Model file for the job. Use its own axes, mm. A direction names the side the tool comes from. Give positions to 0.01 mm unless a question says otherwise; leave off trailing zeros. Loops run counter-clockwise (first coordinate to the right, second up) from the corner with the lowest first, then second, coordinate; pieces in that order, holes last. Notation, with made-up numbers: (-20.75, -33.75) - (24.25, -33.75) arc R22 cw to (24.25, -13.75) - close; hole circle Ø7 at (42, -19.75). An arc over 180 degrees is marked (long way). Use a Markdown table: item, result.
Autodesk Inventor part; units mm, degrees
ref_plane "YZ Plane" through (0, 0, 0) normal (1, 0, 0) x (0, 1, 0)
ref_plane "XZ Plane" through (0, 0, 0) normal (0, 1, 0) x (-1, 0, 0)
ref_plane "XY Plane" through (0, 0, 0) normal (0, 0, 1) x (1, 0, 0)
sketch "Sketch1" plane through (0, 0, 0) normal (0, 0, 1) x (1, 0, 0)
  line L0 (1.5875, 3.175) -> (7.9375, 3.175)
  line L1 (7.9375, 3.175) -> (7.9375, 0)
  line L2 (7.9375, 0) -> (1.5875, 0)
  line L3 (1.5875, 0) -> (1.5875, 3.175)
  line L4 (-7.9375, 3.175) -> (-1.5875, 3.175)
  line L5 (-1.5875, 3.175) -> (-1.5875, 0)
  line L6 (-1.5875, 0) -> (-7.9375, 0)
  line L7 (-7.9375, 0) -> (-7.9375, 3.175)
  line L8 (7.9375, 0) -> (4.7625, 0)
  line L9 (4.7625, 0) -> (4.7625, -3.175)
  line L10 (4.7625, -3.175) -> (7.9375, -3.175)
  line L11 (7.9375, -3.175) -> (7.9375, 0)
  line L12 (-7.9375, 0) -> (-4.7625, 0)
  line L13 (-4.7625, 0) -> (-4.7625, -3.175)
  line L14 (-4.7625, -3.175) -> (-7.9375, -3.175)
  line L15 (-7.9375, -3.175) -> (-7.9375, 0)
  line L16 (-4.7625, -3.175) -> (-1.5875, -6.35)
  line L17 (-1.5875, -6.35) -> (1.5875, -6.35)
  line L18 (1.5875, -6.35) -> (4.7625, -3.175)
  line L19 (7.9375, -3.175) -> (1.5875, -9.525)
  line L20 (1.5875, -9.525) -> (-1.5875, -9.525)
  line L21 (-1.5875, -9.525) -> (-7.9375, -3.175)
  line L22 (-7.9375, -3.175) -> (-4.7625, -3.175)
  point P0 (0, 0)
  dimension "d0" = 6.35
  dimension "d1" = 3.175
  dimension "d2" = 1.5875
  dimension "d3" = 3.175
  dimension "d4" = 6.35
  dimension "d5" = 3.175
  dimension "d6" = 3.175
  dimension "d7" = 4.7625
  dimension "d8" = 4.7625
  dimension "d9" = 3.175
  dimension "d10" = 3.175
  dimension "d11" = 135
  dimension "d12" = 3.175
extrude "Extrusion1" add sketch "Sketch1" against normal blind 50.8
sketch "Sketch2" plane through (7.9375, -3.175, 0) normal (1, 0, 0) x (0, 0, -1)
  line L0 (0, 3.175) -> (50.8, 3.175)
  line L1 (3.175, 3.175) -> (6.35, 3.175)
  line L2 (6.35, 3.175) -> (6.35, -6.35)
  line L3 (6.35, -6.35) -> (3.175, -6.35)
  line L4 (3.175, -6.35) -> (3.175, 3.175)
  line L5 (0, 0) -> (0, 6.35)
  line L6 (9.525, 3.175) -> (12.7, 3.175)
  line L7 (12.7, 3.175) -> (12.7, -6.35)
  line L8 (12.7, -6.35) -> (9.525, -6.35)
  line L9 (9.525, -6.35) -> (9.525, 3.175)
  line L10 (15.875, 3.175) -> (19.05, 3.175)
  line L11 (19.05, 3.175) -> (19.05, -6.35)
  line L12 (19.05, -6.35) -> (15.875, -6.35)
  line L13 (15.875, -6.35) -> (15.875, 3.175)
  line L14 (22.225, 3.175) -> (25.4, 3.175)
  line L15 (25.4, 3.175) -> (25.4, -6.35)
  line L16 (25.4, -6.35) -> (22.225, -6.35)
  line L17 (22.225, -6.35) -> (22.225, 3.175)
  line L18 (28.575, 3.175) -> (31.75, 3.175)
  line L19 (31.75, 3.175) -> (31.75, -6.35)
  line L20 (31.75, -6.35) -> (28.575, -6.35)
  line L21 (28.575, -6.35) -> (28.575, 3.175)
  line L22 (34.925, 3.175) -> (38.1, 3.175)
  line L23 (38.1, 3.175) -> (38.1, -6.35)
  line L24 (38.1, -6.35) -> (34.925, -6.35)
  line L25 (34.925, -6.35) -> (34.925, 3.175)
  line L26 (41.275, 3.175) -> (44.45, 3.175)
  line L27 (44.45, 3.175) -> (44.45, -6.35)
  line L28 (44.45, -6.35) -> (41.275, -6.35)
  line L29 (41.275, -6.35) -> (41.275, 3.175)
  line L30 (47.625, 3.175) -> (50.8, 3.175)
  line L31 (50.8, 3.175) -> (50.8, -6.35)
  line L32 (50.8, -6.35) -> (47.625, -6.35)
  line L33 (47.625, -6.35) -> (47.625, 3.175)
  dimension "d15" = 3.175
  dimension "d16" = 3.175
  dimension "d17" = 9.525
  dimension "d18" = 3.175
  dimension "d19" = 3.175
  dimension "d20" = 3.175
  dimension "d21" = 3.175
  dimension "d22" = 3.175
  dimension "d23" = 3.175
  dimension "d24" = 3.175
  dimension "d25" = 3.175
  dimension "d26" = 3.175
  dimension "d27" = 3.175
  dimension "d28" = 3.175
  dimension "d29" = 3.175
  dimension "d30" = 3.175
  dimension "d31" = 3.175
extrude "Extrusion2" cut sketch "Sketch2" against normal blind 6.35
sketch "Sketch3" plane through (-7.9375, -3.175, 0) normal (-1, 0, 0) x (0, 0, 1)
  line L0 (-3.175, 3.175) -> (-3.175, 3.175)
  line L1 (-50.8, 3.175) -> (-47.625, 3.175)
  line L2 (-47.625, 3.175) -> (-47.625, -6.35)
  line L3 (-47.625, -6.35) -> (-50.8, -6.35)
  line L4 (-50.8, -6.35) -> (-50.8, 3.175)
  line L5 (-44.45, 3.175) -> (-41.275, 3.175)
  line L6 (-41.275, 3.175) -> (-41.275, -6.35)
  line L7 (-41.275, -6.35) -> (-44.45, -6.35)
  line L8 (-44.45, -6.35) -> (-44.45, 3.175)
  line L9 (-38.1, 3.175) -> (-34.925, 3.175)
  line L10 (-34.925, 3.175) -> (-34.925, -6.35)
  line L11 (-34.925, -6.35) -> (-38.1, -6.35)
  line L12 (-38.1, -6.35) -> (-38.1, 3.175)
  line L13 (-31.75, 3.175) -> (-28.575, 3.175)
  line L14 (-28.575, 3.175) -> (-28.575, -6.35)
  line L15 (-28.575, -6.35) -> (-31.75, -6.35)
  line L16 (-31.75, -6.35) -> (-31.75, 3.175)
  line L17 (-25.4, 3.175) -> (-22.225, 3.175)
  line L18 (-22.225, 3.175) -> (-22.225, -6.35)
  line L19 (-22.225, -6.35) -> (-25.4, -6.35)
  line L20 (-25.4, -6.35) -> (-25.4, 3.175)
  line L21 (-19.05, 3.175) -> (-15.875, 3.175)
  line L22 (-15.875, 3.175) -> (-15.875, -6.35)
  line L23 (-15.875, -6.35) -> (-19.05, -6.35)
  line L24 (-19.05, -6.35) -> (-19.05, 3.175)
  line L25 (-12.7, 3.175) -> (-9.525, 3.175)
  line L26 (-9.525, 3.175) -> (-9.525, -6.35)
  line L27 (-9.525, -6.35) -> (-12.7, -6.35)
  line L28 (-12.7, -6.35) -> (-12.7, 3.175)
  line L29 (-6.35, -6.35) -> (-6.35, 3.175)
  line L30 (-6.35, 3.175) -> (-3.175, 3.175)
  line L31 (-3.175, 3.175) -> (-3.175, -6.35)
  line L32 (-3.175, -6.35) -> (-6.35, -6.35)
  point P0 (0, 3.175)
  point P1 (-3.175, 0)
  dimension "d34" = 3.175
  dimension "d35" = 9.525
  dimension "d36" = 3.175
  dimension "d37" = 3.175
  dimension "d38" = 3.175
  dimension "d39" = 3.175
  dimension "d40" = 3.175
  dimension "d41" = 3.175
  dimension "d42" = 3.175
  dimension "d43" = 3.175
  dimension "d44" = 3.175
  dimension "d45" = 3.175
  dimension "d46" = 3.175
  dimension "d47" = 3.175
  dimension "d48" = 3.175
  dimension "d49" = 3.175
extrude "Extrusion3" cut sketch "Sketch3" against normal blind 6.35
sketch "Sketch4" plane through (-7.9375, 3.175, 0) normal (0, 1, 0) x (1, 0, 0)
  circle A0 centre (7.9375, 25.4) radius 9.525
  point P0 (7.9375, 0)
  dimension "d52" = 19.05
extrude "Extrusion4" add sketch "Sketch4" against normal blind 12.7
sketch "Sketch5" plane through (-7.9375, 3.175, 0) normal (0, 1, 0) x (1, 0, 0)
  arc A0 (6.35, 34.7918) -> (6.35, 16.0082) centre (7.9375, 25.4) ccw
  circle A1 centre (7.9375, 25.4) radius 3.4036
  point P0 (7.9375, 0)
  dimension "d55" = 6.8072
extrude "Extrusion5" cut sketch "Sketch5" against normal blind 12.7
sketch "Sketch6" plane through (0, 0, 0) normal (0, 0, 1) x (1, 0, 0)
  line L0 (-1.5875, 3.175) -> (-1.5875, 0)
  line L1 (-1.5875, 3.175) -> (1.5875, 3.175)
  line L2 (1.5875, 3.175) -> (1.5875, -3.175)
  line L3 (1.5875, -3.175) -> (-1.5875, -3.175)
  line L4 (-1.5875, -3.175) -> (-1.5875, 3.175)
  line L5 (-4.7625, -3.175) -> (-4.7625, 0)
  line L6 (-4.7625, 0) -> (4.7625, 0)
  line L7 (4.7625, 0) -> (4.7625, -3.175)
  line L8 (4.7625, -3.175) -> (-4.7625, -3.175)
  line L9 (-4.7625, -3.175) -> (-4.7625, 0)
  point P0 (0, 0)
extrude "Extrusion6" cut sketch "Sketch6" against normal blind 19.05
sketch "Sketch7" plane through (0, 0, -50.8) normal (0, 0, -1) x (-1, 0, 0)
  line L0 (-1.5875, 3.175) -> (-1.5875, 0)
  line L1 (-1.5875, 3.175) -> (1.5875, 3.175)
  line L2 (1.5875, 3.175) -> (1.5875, -3.175)
  line L3 (1.5875, -3.175) -> (-1.5875, -3.175)
  line L4 (-1.5875, -3.175) -> (-1.5875, 3.175)
  line L5 (-4.7625, -3.175) -> (-4.7625, 0)
  line L6 (-4.7625, 0) -> (4.7625, 0)
  line L7 (4.7625, 0) -> (4.7625, -3.175)
  line L8 (4.7625, -3.175) -> (-4.7625, -3.175)
  line L9 (-4.7625, -3.175) -> (-4.7625, 0)
  point P0 (0, 0)
  point P1 (0, 0)
extrude "Extrusion7" cut sketch "Sketch7" against normal blind 19.05
sketch "Sketch9" plane through (0, 0, 0) normal (0, 0, 1) x (1, 0, 0)
  line L0 (4.7625, 0) -> (1.5875, 0)
  line L1 (4.7625, -3.175) -> (4.7625, 0)
  line L2 (4.7625, 0) -> (4.7625, -3.175)
  line L3 (1.5875, -6.35) -> (4.7625, -3.175)
  line L4 (4.7625, -3.175) -> (1.5875, -6.35)
  line L5 (-1.5875, -6.35) -> (1.5875, -6.35)
  line L6 (1.5875, -6.35) -> (-1.5875, -6.35)
  line L7 (-1.5875, -6.35) -> (-4.7625, -3.175)
  line L8 (-1.5875, -6.35) -> (-4.7625, -3.175)
  line L9 (-4.7625, -3.175) -> (-4.7625, 0)
  line L10 (-7.9375, 0) -> (-4.7625, 0)
  line L11 (-4.7625, 0) -> (-7.9375, 0)
  line L12 (-7.9375, 0) -> (-7.9375, -3.175)
  line L13 (-7.9375, -3.175) -> (-1.5875, -9.525)
  line L14 (-7.0995, -4.013) -> (-7.9375, -3.175)
  line L15 (-1.5875, -9.525) -> (1.5875, -9.525)
  line L16 (-1.5875, -9.525) -> (1.5875, -9.525)
  line L17 (7.9375, -3.175) -> (1.5875, -9.525)
  line L18 (1.5875, -9.525) -> (7.9375, -3.175)
  line L19 (7.9375, 0) -> (7.9375, -3.175)
  line L20 (7.9375, -3.175) -> (7.9375, 0)
  line L21 (7.9375, 0) -> (4.7625, 0)
  point P0 (0, 0)
extrude "Extrusion8" add sketch "Sketch9" against normal blind 50.8
sketch "Sketch12" plane through (7.9375, -3.175, 0) normal (1, 0, 0) x (0, 0, -1)
  line L0 (3.175, 3.175) -> (6.35, 3.175)
  line L1 (0, 3.175) -> (19.05, 3.175)
  line L2 (0, 0) -> (17.1511, 0)
  line L3 (6.35, 3.175) -> (3.175, 0)
  line L4 (3.175, 0) -> (3.175, 3.175)
  line L5 (0, 0) -> (0, 6.35)
  line L6 (9.525, 3.175) -> (3.175, -3.175)
  line L7 (3.175, -3.175) -> (6.35, -3.175)
  line L8 (6.35, -3.175) -> (12.7, 3.175)
  line L9 (0, 3.175) -> (19.05, 3.175)
  dimension "d67" = 3.175
properties part number "Basic_rail2"
(1) Slice it at A-A, the plane x = 0. Write the cut outline in (y, z) (3 decimals).
Computed:
| item | result |
|---|---|
| outline | (-9.525, -50.8) - (-6.35, -50.8) - (-6.35, -34.925) - (-3.175, -34.925) - (-3.175, -31.75) - (3.175, -31.75) - (3.175, -28.804) - (-6.35, -28.804) - (-6.35, -21.996) - (3.175, -21.996) - (3.175, -19.05) - (-3.175, -19.05) - (-3.175, -15.875) - (-6.35, -15.875) - (-6.35, 0) - (-9.525, 0) - close |
(2) Mould opens along Z. For faces 1 (the flat face through (-4.762, -2, -9)), 2 (the cylindrical face through (-3.403, -8.804, -25.452)), 3 (the cylindrical face through (-9.523, -4.497, -25.587)) say: pulls with the +Z half, pulls with the -Z half, needs draft (parallel to the pull), parting line crosses it, or undercut.
Computed:
| item | result |
|---|---|
| face 1 | needs draft |
| face 2 | undercut |
| face 3 | parting line crosses it |
(3) Slice it at D-D, the plane x = -6.5. Write the cut outline in (y, z) (1 decimal).
Computed:
| item | result |
|---|---|
| outline | (-9.5, -32.4) - (-4.6, -32.4) - (-4.6, -50.8) - (3.2, -50.8) - (3.2, 0) - (-4.6, 0) - (-4.6, -18.4) - (-9.5, -18.4) - close |
(4) Slice it at B-B, the plane y = -8.5. Count the separate pieces of the cut face and the enclosed holes in it, plus the area to 3 significant figures.
Computed:
| item | result |
|---|---|
| separate pieces | 1 |
| enclosed holes | 2 |
| area | 447 mm² |
(5) 3-axis set-ups, long thin cutter, end or side, ignore diameter. For faces 4 (the flat face through (-3, 0, -9)), 5 (the flat face through (-4.762, -2, -41)), 6 (the flat face through (-2.28, -5.66, -25.36)): which of +Z, -Z, +X, -X, +Y, -Y reach the whole face in a straight line?
Computed:
| item | result |
|---|---|
| face 4 | +Z |
| face 5 | -Z |
| face 6 | +Y |
(6) Drill centre lines: probe 1 along Z at (x, y) = (0, -1.5); probe 2 along X at (y, z) = (2, -32); probe 3 along X at (y, z) = (0.5, -25.4) (3 decimals). Where is each one in solid material? Low to high. Write a range as [from, to].
Computed:
| item | result |
|---|---|
| probe 1 | [-31.75, -28.8], [-22, -19.05] |
| probe 2 | [-7.94, -1.59], [1.59, 7.94] |
| probe 3 | [-9.525, -3.404], [3.404, 9.525] |
(7) Pin check, flat tips, straight feed: P1, Ø1, axis at x = -3.5, z = -12, coming from the -Y side; P2, Ø3.5, axis at x = -0.5, z = -24.5, coming from the +Y side; P3, Ø5, axis at y = 0, z = -10.5, coming from the -X side. Stop position of each tip, or through.
Computed:
| item | result |
|---|---|
| P1 | y = -8.11 |
| P2 | y = -5.69 |
| P3 | x = -7.94 |
